from build123d import *

# Parameters (mm, degrees)
SKETCH1_R           = 2.54
BOSS_EXTRUDE1_DEPTH = 12.7
SKETCH2_W           = 21.59
SKETCH2_H           = 38.1
BOSS_EXTRUDE2_DEPTH = 1.27


with BuildPart() as part:
    # Sketch1 → Boss-Extrude1 (new body)
    with BuildSketch(Plane.XY):
        with BuildLine():
            Line((-31.75, 0), (31.75, 0))
            ThreePointArc((31.75, 0), (38.1, -6.35), (31.75, -12.7))
            Line((31.75, -12.7), (25.4, -12.7))
            Line((25.4, -12.7), (25.4, -38.1))
            Line((25.4, -38.1), (31.75, -38.1))
            ThreePointArc((31.75, -38.1), (38.1, -44.45), (31.75, -50.8))
            Line((31.75, -50.8), (0, -50.8))
            Line((0, -50.8), (-31.75, -50.8))
            ThreePointArc((-31.75, -50.8), (-38.1, -44.45), (-31.75, -38.1))
            Line((-31.75, -38.1), (-25.4, -38.1))
            Line((-25.4, -38.1), (-25.4, -12.7))
            Line((-25.4, -12.7), (-31.75, -12.7))
            ThreePointArc((-31.75, -12.7), (-38.1, -6.35), (-31.75, 0))
        make_face()
        with Locations((-31.75, -6.35)):
            Circle(SKETCH1_R, mode=Mode.SUBTRACT)
        with Locations((31.75, -6.35)):
            Circle(SKETCH1_R, mode=Mode.SUBTRACT)
        with Locations((-31.75, -44.45)):
            Circle(SKETCH1_R, mode=Mode.SUBTRACT)
        with Locations((31.75, -44.45)):
            Circle(SKETCH1_R, mode=Mode.SUBTRACT)
    extrude(amount=BOSS_EXTRUDE1_DEPTH)

    # Sketch2 → Boss-Extrude2 (add)
    with BuildSketch(Plane.XY.offset(12.7)):
        with Locations((0, -19.05)):
            Rectangle(SKETCH2_W, SKETCH2_H)
    extrude(amount=BOSS_EXTRUDE2_DEPTH)


solid = part.part
The listing builds one solid part. Answer for the finished solid, in the listing's coordinates (mm). A direction names the side the tool comes from. Coordinates: 2 decimals unless noted, no trailing zeros. Order: outer loops, then holes, each group sorted by start corner. A loop starts at its lowest first (then second) coordinate and runs counter-clockwise, first axis right, second up.
Q1. Given P1, Ø3, axis at y = -36.5, z = 7.5, coming from the +X side; P2, Ø6.5, axis at x = -31.75, y = -6.35, coming from the +Z side; P3, Ø4.5, axis at x = -31.75, y = -44.45, coming from the -Z side; P4, Ø8, axis at y = -18.5, z = 2, coming from the -X side, each flat-ended and moving along its own axis, determine where each tip first touches the part or whether it passes through.
Q2. A cutting plane is placed at C-C, the plane z = 9.75. Write down the section's boundary in (x, y), and give its area (3 significant figures).
Q3. A cutting plane is placed at D-D, the plane y = -18.5. Write down the section's boundary in (x, z) (3 decimals), and give its area (3 significant figures).
Q4. For a pull along Y with two mould halves and no side action, classify faces 4 (the face through (-29, -12.7, 6)), 5 (the face through (0, 0, 7)), 6 (the face through (1, -25, 0)) as pulls with the +Y half, pulls with the -Y half, needs draft (parallel to the pull), parting line crosses it, or undercut.
Q5. Which of the six approach directions +Z, -Z, +X, -X, +Y, -Y give full straight-line access (tool end or side, diameter ignored) to faces 1 (the face through (31.2, -46.93, 6.26)), 2 (the face through (29, -12.7, 6)), 3 (the face through (-25.4, -26, 6))?
Q6. Consider line 1 (Y direction, x = -31.5, z = 10.5); line 2 (Y direction, x = 31, z = 4.5); line 3 (X direction, y = -43.5, z = 5.25). Determine where each line is inside the solid, lowest interval first.
Q7. A cutting plane is placed at A-A, the plane y = -6.35. Write down the section's boundary in (x, z) (3 decimals), and give its area (3 significant figures).
Q8. A cutting plane is placed at B-B, the plane x = 28. Write down the section's boundary in (y, z), and give its area (3 significant figures).
Answers follow:
1. P1: stops at x = 25.4
1. P2: stops at z = 12.7
1. P3: passes through
1. P4: stops at x = -25.4
2. outline: (-31.75, -50.8) - (31.75, -50.8) arc R6.35 ccw to (31.75, -38.1) - (25.4, -38.1) - (25.4, -12.7) - (31.75, -12.7) arc R6.35 ccw to (31.75, 0) - (-31.75, 0) arc R6.35 ccw to (-31.75, -12.7) - (-25.4, -12.7) - (-25.4, -38.1) - (-31.75, -38.1) arc R6.35 ccw to start; hole circle Ø5.08 at (-31.75, -44.45); hole circle Ø5.08 at (-31.75, -6.35); hole circle Ø5.08 at (31.75, -44.45); hole circle Ø5.08 at (31.75, -6.35)
2. area: 3,080 mm2
3. outline: (-25.4, 0) - (25.4, 0) - (25.4, 12.7) - (10.795, 12.7) - (10.795, 13.97) - (-10.795, 13.97) - (-10.795, 12.7) - (-25.4, 12.7) - close
3. area: 673 mm2
4. face 4: undercut
4. face 5: pulls with the +Y half
4. face 6: needs draft
5. face 1: +Z, -Z
5. face 2: +Z, -Z, +X
5. face 3: +Z, -Z, -X
6. line 1: y = -50.8 to -46.98, -41.92 to -38.1, -12.7 to -8.88, -3.82 to 0
6. line 2: y = -50.8 to -46.88, -42.02 to -38.1, -12.7 to -8.78, -3.92 to 0
6. line 3: x = -38.03 to -34.11, -29.39 to 29.39, 34.11 to 38.03
7. outline: (-38.1, 0) - (-34.29, 0) - (-34.29, 12.7) - (-38.1, 12.7) - close; (-29.21, 0) - (29.21, 0) - (29.21, 12.7) - (10.795, 12.7) - (10.795, 13.97) - (-10.795, 13.97) - (-10.795, 12.7) - (-29.21, 12.7) - close; (34.29, 0) - (38.1, 0) - (38.1, 12.7) - (34.29, 12.7) - close
7. area: 866 mm2
8. outline: (-50.8, 0) - (-38.1, 0) - (-38.1, 12.7) - (-50.8, 12.7) - close; (-12.7, 0) - (0, 0) - (0, 12.7) - (-12.7, 12.7) - close
8. area: 323 mm2
